```python
from build123d import *

# Parameters (mm, degrees)
SKETCH1_R               = 1.2295
BASENUT_DEPTH           = 2.4
ENDCHAMFER_SIZE         = 0.2705
ENDCHAMFER_SIZE2        = 0.156173248
ENDCHAMFER_PART_2_SIZE  = 0.2705
ENDCHAMFER_PART_2_SIZE2 = 0.156173248


with BuildPart() as part:
    # Sketch1 → BaseNut (new body)
    with BuildSketch(Plane.XY):
        Polygon((3.175426481, 0), (1.58771324, 2.75), (-1.58771324, 2.75), (-3.175426481, 0), (-1.58771324, -2.75), (1.58771324, -2.75), align=None)
        Circle(SKETCH1_R, mode=Mode.SUBTRACT)
    extrude(amount=-BASENUT_DEPTH)

    # Sketch2 → Double-Chamfer (revolve, cut)
    with BuildSketch(Plane(origin=(0, 0, 0), x_dir=(1, 0, 0), z_dir=(0, 1, 0))):
        Polygon((-3.175426481, 2.4), (-2.375, 2.4), (-3.175426481, 1.937873556), align=None)
        Polygon((-3.175426481, 0.462126444), (-3.175426481, 0), (-2.375, 0), align=None)
    revolve(axis=Axis((0, 0, -3.375940562), (0, 0, 1)), mode=Mode.SUBTRACT)

    # EndChamfer
    endchamfer_edges = [part.edges().sort_by_distance(p)[0] for p in [
        (-1.2295, 0, -2.4),
    ]]
    endchamfer_side = [part.faces().sort_by_distance(p)[0] for p in [
        (-1.2295, 0, -1.2),
    ]]
    chamfer(endchamfer_edges, length=ENDCHAMFER_SIZE, length2=ENDCHAMFER_SIZE2, reference=endchamfer_side[0])

    # EndChamfer part 2
    endchamfer_part_2_edges = [part.edges().sort_by_distance(p)[0] for p in [
        (-1.2295, 0, 0),
    ]]
    endchamfer_part_2_side = [part.faces().sort_by_distance(p)[0] for p in [
        (2.307824856, 0, 0),
    ]]
    chamfer(endchamfer_part_2_edges, length=ENDCHAMFER_PART_2_SIZE, length2=ENDCHAMFER_PART_2_SIZE2, reference=endchamfer_part_2_side[0])


solid = part.part
```
Design review of the part built by this model. Coordinates are the model's own, in mm. Give positions to 0.01 mm unless a question says otherwise; leave off trailing zeros. Order: outer loops, then holes, each group sorted by start corner. A loop starts at its lowest first (then second) coordinate and runs counter-clockwise, first axis right, second up. Notation, with made-up numbers: (8.5, 37) -> (51.5, 37) arc R21 ccw to (51.5, 64) -> close; hole circle Ø3 at (-38.75, 66.25). An arc over 180 degrees is marked (long way). Write item = value, one per line. Start each with the question number.
(1) Mouldability with a two-part tool opening along X and no side actions: class faces 1 (the face through (2.37, -1.394, -1.186)), 2 (the face through (-0.976, -0.748, -1.129)), 3 (the face through (-2.37, 1.394, -1.186)), 4 (the face through (0, 2.75, -1)) as +X half, -X half, draft (parallel to the pull), parting line (faces both ways), or undercut.
(2) We need section B-B on z = -0.3. Write out the cut boundary in (x, y).
(3) To check wall thickness, follow line 1 along Y through (x, z) = (0, -1.25); line 2 along X through (y, z) = (0.5, -0.4); line 3 along X through (y, z) = (-1.05, -0.8). State the ranges of each line that lie inside material, in increasing order.
(4) For pin 1 (1 mm diameter, centred on y = -1.5, z = -0.5, fed in from +X); pin 2 (1 mm diameter, centred on x = 1.5, z = -2, fed in from -Y), all flat-tipped, find the tip position at first contact; note any pin that passes through.
Numbers:
q1.face_1 = +X half
q1.face_2 = undercut
q1.face_3 = -X half
q1.face_4 = draft
q2.outline = (-2.83, -0.59) -> (-1.93, -2.16) arc R2.89 ccw to (-0.9, -2.75) -> (0.9, -2.75) arc R2.89 ccw to (1.93, -2.16) -> (2.83, -0.59) arc R2.89 ccw to (2.83, 0.59) -> (1.93, 2.16) arc R2.89 ccw to (0.9, 2.75) -> (-0.9, 2.75) arc R2.89 ccw to (-1.93, 2.16) -> (-2.83, 0.59) arc R2.89 ccw to start; hole circle Ø2.46 at (0, 0)
q3.line_1 = -2.75 to -1.23, 1.23 to 2.75
q3.line_2 = -2.89 to -1.12, 1.12 to 2.89
q3.line_3 = -2.57 to -0.64, 0.64 to 2.57
q4.pin_1 = 2.6
q4.pin_2 = -2.75
